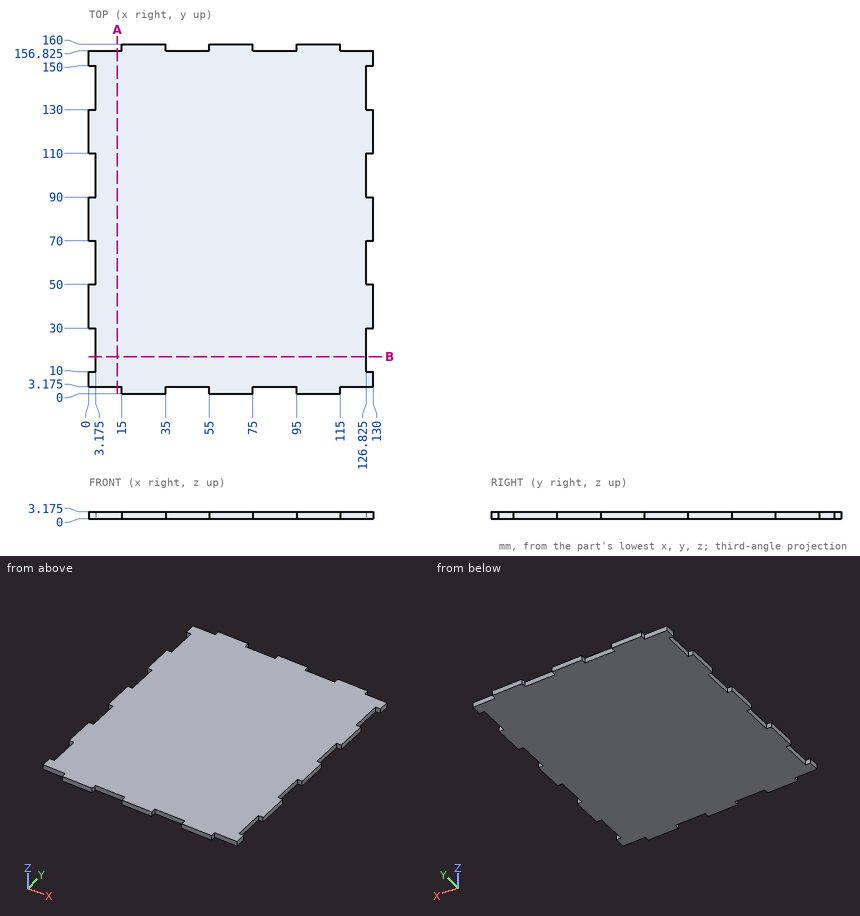
Print and shaded views of the part. All mm, measured from the part's lowest x, y and z. Coordinates: 2 decimals unless noted, no trailing zeros. Order: outer loops, then holes, each group sorted by start corner. A loop starts at its lowest first (then second) coordinate and runs counter-clockwise, first axis right, second up. Notation, with made-up numbers: M 69,31.5 L 83,31.5 A24 cw 83,60.5 Z; hole C 40,8 d7. An arc over 180 degrees is marked long. Answer as CSV lines item,"result".
1) Drill centre lines: L1, parallel to X at y = 105, z = 2.45 (3 decimals); L2, parallel to Y at x = 122.5, z = 3.05 (3 decimals). Where is each one in solid material? Low to high. Write a range as from..to.
Verdict:
L1,"3.175..126.825"
L2,"3.175..156.825"
2) Cut at A-A (x = 13). List the corners of the cut face in (y, z) (3 decimals), then the cut area to 3 significant figures.
Verdict:
outline,"M 3.175,0 L 156.825,0 L 156.825,3.175 L 3.175,3.175 Z"
area,"488 mm2"
3) Cut at B-B (y = 17). List the corners of the cut face in (x, z) (3 decimals), then the cut area to 3 significant figures.
Verdict:
outline,"M 3.175,0 L 126.825,0 L 126.825,3.175 L 3.175,3.175 Z"
area,"393 mm2"
4) Flat gauge pins, fed straight in: P1, Ø1, axis at y = 159, z = 1.5, coming from the +X side; P2, Ø1.6, axis at x = 129, z = 2.5, coming from the -Y side (3 decimals); P3, Ø1.5, axis at y = 67.5, z = 3, coming from the +X side (3 decimals). Where does each tip first touch, or does it go through?
Verdict:
P1,"x = 115"
P2,"y = 3.175"
P3,"x = 126.825"
